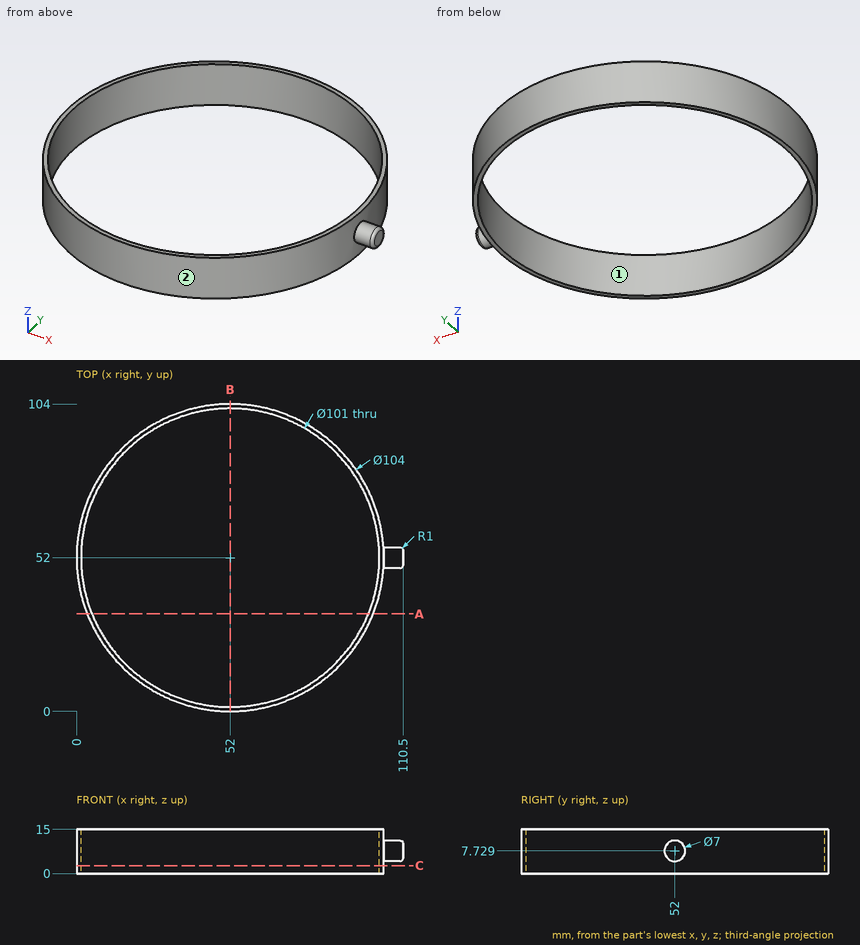
Job drawing, mm, ordinate dimensions from the low corner. One solid piece. Coordinates: 2 decimals unless noted, no trailing zeros. Order: outer loops, then holes, each group sorted by start corner. A loop starts at its lowest first (then second) coordinate and runs counter-clockwise, first axis right, second up. Notation, with made-up numbers: (43, -33.5) - (58, -33.5) arc R19 cw to (58, -16.5) - close; hole circle Ø4 at (55, 46.25). An arc over 180 degrees is marked (long way). Return JSON: item names as keys, results as strings. Group by question number.
1) Saw through at C-C, the plane z = 2.75. Write the cut outline in (x, y), plus the area to 3 significant figures.
2) Probe line 1 (X direction, y = 50.5, z = 5.5); line 2 (Y direction, x = 52, z = 8.5); line 3 (X direction, y = 22, z = 7.5). List the from-to ranges inside material, lowest first. Write a range as from..to.
3) Mould opens along Y. For the marked faces 1 and 2 say: released by +Y, released by -Y, zero draft, split by the parting line, or undercut.
4) Flat gauge pins, fed straight in: P1, Ø6, axis at y = 41, z = 13.5, coming from the -X side; P2, Ø4, axis at x = 24, z = 13.5, coming from the -Y side; P3, Ø2, axis at x = 59.5, z = 11.5, coming from the -Y side. Where does each tip first touch, or does it go through?
5) Saw through at B-B, the plane x = 52. Write the cut outline in (y, z), plus the area to 3 significant figures.
6) Saw through at A-A, the plane y = 33. Write the cut outline in (x, z).
Values found:
{
 "1": {"outline": "circle Ø104 at (52, 52); hole circle Ø101 at (52, 52)", "area": "483 mm²"},
 "2": {"line 1": "x = 0.02..1.52, 102.48..110.48", "line 2": "y = 0..1.5, 102.5..104", "line 3": "x = 9.53..11.38, 92.62..94.47"},
 "3": {"face 1": "undercut", "face 2": "split by the parting line"},
 "4": {"P1": "stops at x = 0.62", "P2": "stops at y = 6.97", "P3": "stops at y = 0.41"},
 "5": {"outline": "(0, 0) - (1.5, 0) - (1.5, 15) - (0, 15) - close; (102.5, 0) - (104, 0) - (104, 15) - (102.5, 15) - close", "area": "45.0 mm²"},
 "6": {"outline": "(3.6, 0) - (5.21, 0) - (5.21, 15) - (3.6, 15) - close; (98.79, 0) - (100.4, 0) - (100.4, 15) - (98.79, 15) - close"}
}
